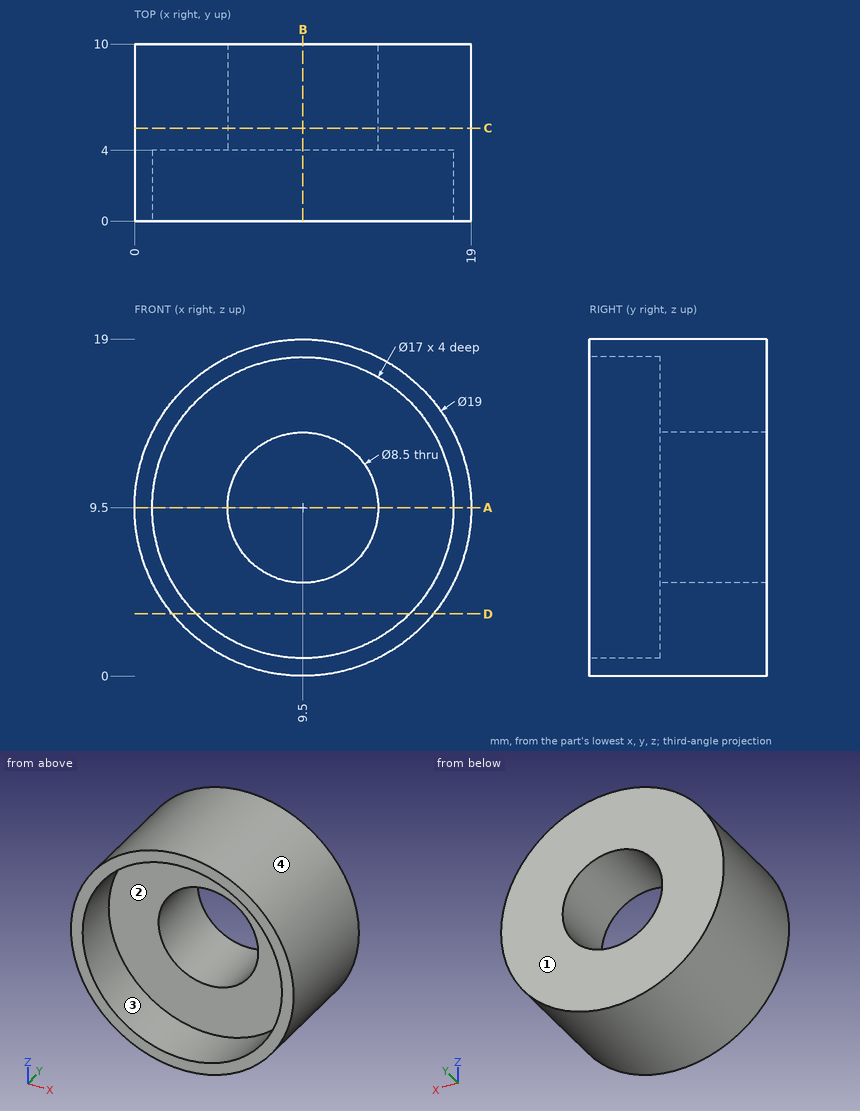
Study the drawing (mm; zero at the part's minimum x, y, z) and answer. Coordinates: 2 decimals unless noted, no trailing zeros. Write each loop counter-clockwise with the first axis right and the second up, starting at its lowest first coordinate (ties: lowest second). Pieces come first, ordered by that corner, then holes. Notation, with made-up numbers: (31.25, 59) -> (78.25, 59) arc R21 cw to (78.25, 94) -> close; hole circle Ø11 at (59, 77). An arc over 180 degrees is marked (long way). Write item = value, one per line.
(1) Straight lines are drawn through the part: L1, parallel to Z at x = 9.5, y = 8.1; L2, parallel to X at y = 2.35, z = 9.5. For each, find the intervals that lie inside material, in ascending order. Write a range as from..to.
From the geometry:
L1 = 0..5.25, 13.75..19
L2 = 0..1, 18..19
(2) Given pin 1 Ø1 at (x, y) = (12.5, 6) entering from -Z; pin 2 Ø5 at (x, z) = (10, 5.5) entering from -Y; pin 3 Ø1.5 at (y, z) = (2, 6.5) entering from +X, each flat-ended and moving along its own axis, determine where each tip first touches the part or whether it passes through.
From the geometry:
pin_1 = 0.33
pin_2 = 4
pin_3 = 18.73
(3) Section C-C on y = 5.25 is taken. Write down the section's boundary in (x, z), plus the area to 3 significant figures.
From the geometry:
outline = circle Ø19 at (9.5, 9.5); hole circle Ø8.5 at (9.5, 9.5)
area = 227 mm2
(4) Section D-D on z = 3.5 is taken. Write down the section's boundary in (x, y), plus the area to 3 significant figures.
From the geometry:
outline = (2.13, 0) -> (3.48, 0) -> (3.48, 4) -> (15.52, 4) -> (15.52, 0) -> (16.87, 0) -> (16.87, 10) -> (2.13, 10) -> close
area = 99.1 mm2
(5) Section A-A on z = 9.5 is taken. Write down the section's boundary in (x, y), plus the area to 3 significant figures.
From the geometry:
outline = (0, 0) -> (1, 0) -> (1, 4) -> (5.25, 4) -> (5.25, 10) -> (0, 10) -> close; (13.75, 4) -> (18, 4) -> (18, 0) -> (19, 0) -> (19, 10) -> (13.75, 10) -> close
area = 71.0 mm2
(6) For a pull along Z with two mould halves and no side action, classify the marked faces 1, 2, 3 and 4 as +Z half, -Z half, draft (parallel to the pull), parting line (faces both ways), or undercut.
From the geometry:
face_1 = draft
face_2 = undercut
face_3 = undercut
face_4 = parting line
(7) Section B-B on x = 9.5 is taken. Write down the section's boundary in (y, z).
From the geometry:
outline = (0, 0) -> (10, 0) -> (10, 5.25) -> (4, 5.25) -> (4, 1) -> (0, 1) -> close; (0, 18) -> (4, 18) -> (4, 13.75) -> (10, 13.75) -> (10, 19) -> (0, 19) -> close
